```python
from build123d import *

# Parameters (mm, degrees)
F0_W     = 127
F0_H     = 76.2
F1_DEPTH = 50.8
F2_R     = 24.309053
F3_DEPTH = 50.801
F4_T     = -2.54
F5_R     = 6.35


with BuildPart() as f1:
    # F0 (on Top) → F1 (new body)
    with BuildSketch(Plane.XY):
        with Locations((63.5, 38.1)):
            Rectangle(F0_W, F0_H)
    extrude(amount=F1_DEPTH)

    # F2 (on face) → F3 (cut, through all)
    with BuildSketch(Plane.XY.offset(50.8)):
        with Locations((36.587957, 47.760736)):
            Circle(F2_R)
    extrude(amount=-F3_DEPTH, mode=Mode.SUBTRACT)

    # F4
    f4_openings = [f1.faces().sort_by_distance(p)[0] for p in [
        (12.278904, 47.760736, 25.4),
    ]]
    offset(amount=F4_T, openings=f4_openings)

    # F5
    f5_edges = [f1.edges().sort_by_distance(p)[0] for p in [
        (127, 76.2, 25.4),
        (127, 38.1, 0),
        (127, 0, 25.4),
        (127, 38.1, 50.8),
    ]]
    fillet(f5_edges, radius=F5_R)


solid = f1.part
```
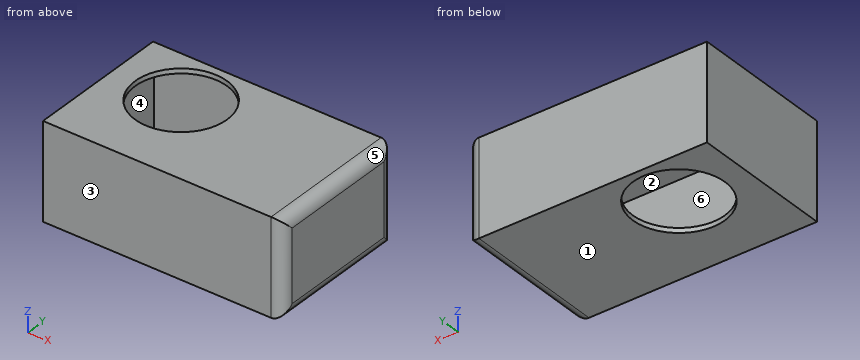
Can you work these out from the model? Positions are in its coordinate system, mm. Face numbers are marked on the shaded views. A direction names the side the tool comes from. Round coordinates to 2 decimals unless told otherwise and drop trailing zeros. Loops run counter-clockwise (first coordinate to the right, second up) from the corner with the lowest first, then second, coordinate; pieces in that order, holes last. Notation, with made-up numbers: (40, 43) -> (51, 43) arc R23 ccw to (51, 77) -> close; hole circle Ø9 at (-22.75, -35.75). An arc over 180 degrees is marked (long way). One line per item, written item: value. Start each with the question number.
1. If we mould it in two halves opening along Z, with no side actions, what happens to the marked faces 3, 4, 5 and 6? For each: pulls with the +Z half, pulls with the -Z half, needs draft (parallel to the pull), parting line crosses it, or undercut.
2. For the marked faces 1 and 2, which set-ups out of +Z, -Z, +X, -X, +Y, -Y let a thin tool reach every point of the face, with its end or its side?
3. If I drill on probe 1 along X at (y, z) = (48, 8.5); probe 2 along Z at (x, y) = (74.5, 54.5); probe 3 along Y at (x, z) = (81.5, 14), over which ranges is the centre line in solid material (lowest first)?
4. If we section it at B-B, the plane y = 34: Write out the boundary of the cut face in (x, z), then the cut area to 3 significant figures.
5. For pin 1 (2 mm diameter, centred on x = 64, z = 12, fed in from -Y), with a flat end and sliding along its axis, tell me the tip position at first contact or that it passes through.
6. If we section it at C-C, the plane z = 20: Write out the boundary of the cut face in (x, y).
7. If we section it at D-D, the plane x = 27.5: Write out the boundary of the cut face in (y, z), then the cut area to 3 significant figures.
8. If we section it at A-A, the plane x = 110.5: Write out the boundary of the cut face in (y, z), then the cut area to 3 significant figures.
Calculated:
1. face 3: needs draft
1. face 4: undercut
1. face 5: pulls with the +Z half
1. face 6: undercut
2. face 1: -Z, +X, -X, +Y, -Y
2. face 2: none
3. probe 1: x = 0 to 2.54, 124.46 to 127
3. probe 2: z = 0 to 2.54, 48.26 to 50.8
3. probe 3: y = 0 to 2.54, 73.66 to 76.2
4. outline: (0, 0) -> (16.55, 0) -> (16.55, 2.54) -> (2.54, 2.54) -> (2.54, 48.26) -> (16.55, 48.26) -> (16.55, 50.8) -> (0, 50.8) -> close; (56.63, 0) -> (120.65, 0) arc R6.35 ccw to (127, 6.35) -> (127, 44.45) arc R6.35 ccw to (120.65, 50.8) -> (56.63, 50.8) -> (56.63, 48.26) -> (124.46, 48.26) -> (124.46, 2.54) -> (56.63, 2.54) -> close
4. area: 657 mm²
5. pin 1: stops at y = 0
6. outline: (0, 0) -> (120.65, 0) arc R6.35 ccw to (127, 6.35) -> (127, 69.85) arc R6.35 ccw to (120.65, 76.2) -> (0, 76.2) -> close; hole (2.54, 2.54) -> (124.46, 2.54) -> (124.46, 73.66) -> (2.54, 73.66) -> close
7. outline: (0, 0) -> (25.21, 0) -> (25.21, 2.54) -> (2.54, 2.54) -> (2.54, 48.26) -> (25.21, 48.26) -> (25.21, 50.8) -> (0, 50.8) -> close; (70.31, 0) -> (76.2, 0) -> (76.2, 50.8) -> (70.31, 50.8) -> (70.31, 48.26) -> (73.66, 48.26) -> (73.66, 2.54) -> (70.31, 2.54) -> close
7. area: 390 mm²
8. outline: (0, 0) -> (76.2, 0) -> (76.2, 50.8) -> (0, 50.8) -> close; hole (2.54, 2.54) -> (73.66, 2.54) -> (73.66, 48.26) -> (2.54, 48.26) -> close
8. area: 619 mm²
